Here's how the part is built. I have some questions about the finished solid (model axes, mm). Face numbers are marked on the shaded views. A direction names the side the tool comes from. Give positions to 0.01 mm unless a question says otherwise; leave off trailing zeros. Loops run counter-clockwise (first coordinate to the right, second up) from the corner with the lowest first, then second, coordinate; pieces in that order, holes last. Notation, with made-up numbers: M -25.75,-35.5 L 20.25,-35.5 A28 ccw 20.25,-17.5 Z; hole C -26.5,70 d8. An arc over 180 degrees is marked long. Answer as CSV lines item,"result". Start each with the question number.
Item 1: For the marked faces 1 and 2, which set-ups out of +Z, -Z, +X, -X, +Y, -Y let a thin tool reach every point of the face, with its end or its side?
Item 2: Will these pins go through, and if not, where does the flat tip stop? P1, Ø10, axis at x = 12, z = 28.5, coming from the -Y side; P2, Ø5, axis at x = 7, z = 24.5, coming from the -Y side; P3, Ø3, axis at y = -14.5, z = 24.5, coming from the -X side.
Item 3: If I drill on line 1 along X through (y, z) = (-22.75, 28.5); line 2 along Z through (x, y) = (2.5, -15.5); line 3 along Y through (x, z) = (13, 21), over which ranges is the centre line in solid material (lowest first)? Write a range as from..to.
Item 4: I want a section at B-B on x = 15. List the corners of the cut face in (y, z) for me.
Item 5: I want a section at A-A on y = -20.75. List the corners of the cut face in (x, z) for me.
Item 6: I want a section at C-C on z = 12.5. List the corners of the cut face in (x, y) for me.
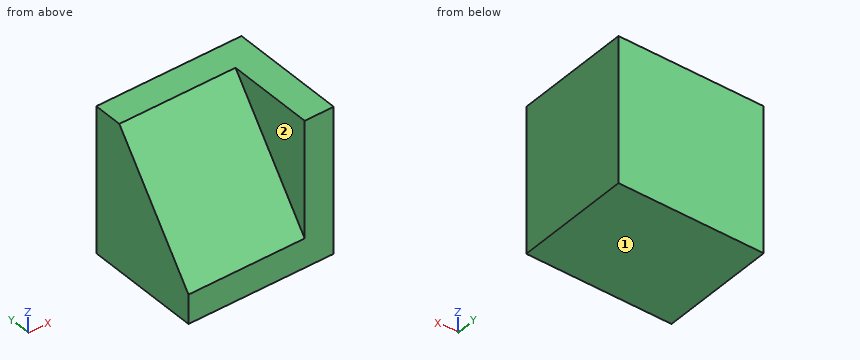
from build123d import *

# Parameters (mm, degrees)
F0_W     = 31.75
F0_H     = 31.75
F1_DEPTH = 25.4
F3_DEPTH = 25.4


with BuildPart() as f1:
    # F0 (on Front) → F1 (new body)
    with BuildSketch(Plane.XZ):
        with Locations((15.875, 15.875)):
            Rectangle(F0_W, F0_H)
    extrude(amount=F1_DEPTH)

    # F2 (on Right) → F3 (cut)
    with BuildSketch(Plane.YZ):
        Polygon((-25.4, 6.35), (-6.35, 31.75), (-25.4, 31.75), align=None)
    extrude(amount=F3_DEPTH, mode=Mode.SUBTRACT)


solid = f1.part
Result:
1,face 1,"-Z, +X, -X, +Y, -Y"
1,face 2,"+Z, -X, -Y"
2,P1,"y = -12.54"
2,P2,"y = -13.66"
2,P3,"x = 25.4"
3,line 1,"25.4..31.75"
3,line 2,"0..19.55"
3,line 3,"-14.41..0"
4,outline,"M -25.4,0 L 0,0 L 0,31.75 L -6.35,31.75 L -25.4,6.35 Z"
5,outline,"M 0,0 L 31.75,0 L 31.75,31.75 L 25.4,31.75 L 25.4,12.55 L 0,12.55 Z"
6,outline,"M 0,-20.79 L 25.4,-20.79 L 25.4,-25.4 L 31.75,-25.4 L 31.75,0 L 0,0 Z"
